Part model, mm, in its own coordinate system. A direction names the side the tool comes from. Coordinates: 2 decimals unless noted, no trailing zeros. Loops run counter-clockwise (first coordinate to the right, second up) from the corner with the lowest first, then second, coordinate; pieces in that order, holes last. Notation, with made-up numbers: M 71.5,49.25 L 127.5,49.25 A16 cw 127.5,56.25 Z; hole C 43.5,65.5 d6. An arc over 180 degrees is marked long. Use a Markdown table: item, result. Add a question column.
1) Wall check: probe 1 along Y at (x, z) = (2, 5.75); probe 2 along X at (y, z) = (9.5, 8.75); probe 3 along X at (y, z) = (7, 7). Give the ranges that are in metal, low to high. Write a range as from..to.
2) Band-saw the part on B-B (x = 3.25). List the corners of the cut face in (y, z), plus the area to 3 significant figures.
3) Pull direction Y, two halves, no side cores. Call faces 1 (the cylindrical face through (7.495, 18.161, 4.437)), 2 (the flat face through (3, 0, 4)), 3 (the cylindrical face through (3.85, -27.4, 4.44)), 4 (the cylindrical face through (0.285, 9.619, 8.699)): released by +Y, released by -Y, zero draft, split by the parting line, or undercut.
4) Tool access for faces 5 (the cylindrical face through (8.676, -6.765, 4.437)), 6 (the cylindrical face through (3.028, 0.285, 0.301)), 7 (the cylindrical face through (3.028, 0.285, 8.699)), 8 (the cylindrical face through (3.7, 18.6, 8.8)), 9 (the cylindrical face through (0.285, 18.699, 4.549)): list every direction of +Z, -Z, +X, -X, +Y, -Y with a clear straight run to the whole face (end or side of a thin tool).
5) Pin check, flat tips, straight feed: pin 1 Ø2.5 at (y, z) = (5, 6.5) entering from +X; pin 2 Ø1.2 at (x, z) = (3.5, 3) entering from -Y; pin 3 Ø2 at (y, z) = (-0.5, 7.5) entering from -X. Stop position of each tip, or through.
6) Band-saw the part on A-A (z = 7). List the corners of the cut face in (x, y).
from build123d import *

# Parameters (mm, degrees)
PAD_DEPTH = 9
FILLET_R  = 1


with BuildPart() as part:
    # Sketch → Pad (new body)
    with BuildSketch(Plane.XY):
        with BuildLine():
            Line((0, 0), (0, 19))
            Line((0, 19), (5, 19))
            ThreePointArc((9.791817, 17.032919), (7.461019, 18.175071), (5, 19))
            ThreePointArc((6.222729, -29.25408), (11.317567, -6.36583), (9.791817, 17.032919))
            ThreePointArc((5, -24.689043), (3.859753, -27.440724), (6.222729, -29.25408))
            ThreePointArc((5, -24.689043), (8.692964, -6.505033), (7.329164, 12))
            ThreePointArc((7.329164, 12), (6.164582, 13.164582), (5, 12))
            Line((5, 0), (5, 12))
            Line((0, 0), (5, 0))
        make_face()
    extrude(amount=PAD_DEPTH)

    # Fillet
    fillet_edges = [part.edges().sort_by_distance(p)[0] for p in [
        (0, 0, 4.5),
        (0, 19, 4.5),
        (0, 9.5, 0),
        (0, 9.5, 9),
        (2.5, 19, 9),
        (2.5, 19, 0),
        (2.5, 0, 0),
        (2.5, 0, 9),
        (11.317567, -6.36583, 9),
        (11.317567, -6.36583, 0),
    ]]
    fillet(fillet_edges, radius=FILLET_R)


solid = part.part
Entries:
| question | item | result |
|---|---|---|
| 1 | probe 1 | 0..19 |
| 1 | probe 2 | 0.34..5, 7.81..10.68 |
| 1 | probe 3 | 0..5, 8.2..11.27 |
| 2 | outline | M 0,1 A1 ccw 1,0 L 18,0 A1 ccw 19,1 L 19,8 A1 ccw 18,9 L 1,9 A1 ccw 0,8 Z |
| 2 | area | 170 mm2 |
| 3 | face 1 | released by +Y |
| 3 | face 2 | undercut |
| 3 | face 3 | undercut |
| 3 | face 4 | zero draft |
| 4 | face 5 | +Z, -Z |
| 4 | face 6 | -Z, -X |
| 4 | face 7 | +Z, -X |
| 4 | face 8 | +Z, +X, -X, +Y |
| 4 | face 9 | +Z, -Z, -X, +Y |
| 5 | pin 1 | x = 11.48 |
| 5 | pin 2 | y = -28.02 |
| 5 | pin 3 | x = 0.13 |
| 6 | outline | M 0,1 A1 ccw 1,0 L 5,0 L 5,12 A1.16 cw 7.33,12 A67.95 cw 5,-24.69 A2.45 ccw 6.22,-29.25 A82.8 ccw 9.79,17.03 A19.65 ccw 5,19 L 1,19 A1 ccw 0,18 Z |
